Check sheet for the modelled part. Datum: model origin and axes. Units: mm. Round coordinates to 2 decimals unless told otherwise and drop trailing zeros. Order: outer loops, then holes, each group sorted by start corner. A loop starts at its lowest first (then second) coordinate and runs counter-clockwise, first axis right, second up. Notation, with made-up numbers: M 7.25,81.25 L 53.25,81.25 A34 cw 53.25,120.25 Z; hole C 72.5,33 d10. An arc over 180 degrees is marked long. One line per item, written item: value. Start each with the question number.
(1) Thickness scan on L1, parallel to Y at x = -15.5, z = 0.55; L2, parallel to Y at x = 15.5, z = 1.35; L3, parallel to X at y = -2.25, z = 0.1. Record the ranges inside material, lowest first.
(2) Cross-section at C-C, the plane y = -4. Enter the section's corners in (x, z).
(3) Release check for a two-part mould opening along Y. For faces 1 (the face through (0, 0, 0)), 2 (the face through (-18.347, -0.125, 0.592)), 3 (the face through (0, -4.5, 1)), 4 (the face through (17.169, -0.526, 0.986)) record: released by +Y, released by -Y, zero draft, split by the parting line, or undercut.
(4) Cross-section at A-A, the plane y = 0. Enter the section's corners in (x, z).
(5) Cross-section at B-B, the plane z = 1.6. Enter the section's corners in (x, y), and give its area (3 significant figures).
Autodesk Inventor part; units mm, degrees
ref_plane "YZ Plane" through (0, 0, 0) normal (1, 0, 0) x (0, 1, 0)
ref_plane "XZ Plane" through (0, 0, 0) normal (0, 1, 0) x (-1, 0, 0)
ref_plane "XY Plane" through (0, 0, 0) normal (0, 0, 1) x (1, 0, 0)
sketch "Sketch1" plane through (0, 0, 0) normal (0, 0, 1) x (1, 0, 0)
  line L0 (-15.5, 0) -> (15.5, 0) construction
  line L1 (-15.5, -4.5) -> (15.5, -4.5)
  line L2 (15.5, 4.5) -> (-15.5, 4.5)
  arc A0 (-15.5, 4.5) -> (-15.5, -4.5) centre (-15.5, 0) ccw
  arc A1 (15.5, -4.5) -> (15.5, 4.5) centre (15.5, 0) ccw
  circle A2 centre (-15.5, 0) radius 2.85
  circle A3 centre (15.5, 0) radius 1.75
  point P0 (0, 0)
  point P1 (0, 0)
  dimension "d0" = 9
  dimension "d1" = 31
  dimension "d2" = 5.7
  dimension "d3" = 3.5
extrude "Extrusion1" add sketch "Sketch1" along normal blind 2
chamfer "Chamfer1" distance 0.8 angle 45 1 edges at (-18.35, 0, 2)
properties part number "gripper_mechanism2"
Values found:
1. L1: -4.5 to -2.85, 2.85 to 4.5
1. L2: -4.5 to -1.75, 1.75 to 4.5
1. L3: -19.4 to -17.25, -13.75 to 19.4
2. outline: M -17.56,0 L 17.56,0 L 17.56,2 L -17.56,2 Z
3. face 1: zero draft
3. face 2: undercut
3. face 3: released by -Y
3. face 4: undercut
4. outline: M -20,0 L -18.35,0 L -18.35,1.2 L -19.15,2 L -20,2 Z; M -12.65,0 L 13.75,0 L 13.75,2 L -11.85,2 L -12.65,1.2 Z; M 17.25,0 L 20,0 L 20,2 L 17.25,2 Z
5. outline: M -15.5,-4.5 L 15.5,-4.5 A4.5 ccw 15.5,4.5 L -15.5,4.5 A4.5 ccw Z; hole C -15.5,0 d6.5; hole C 15.5,0 d3.5
5. area: 300 mm^2
